Design review of the part shown in the three views and the two pictorial views. Dimensions are in mm from the part's minimum x, y and z. Round coordinates to 2 decimals unless told otherwise and drop trailing zeros. Loops run counter-clockwise (first coordinate to the right, second up) from the corner with the lowest first, then second, coordinate; pieces in that order, holes last. Notation, with made-up numbers: (-29.75, 33) -> (6.25, 33) arc R20 cw to (6.25, 55) -> close; hole circle Ø11 at (-2, 30.5). An arc over 180 degrees is marked (long way). Return JSON: item names as keys, results as strings. Group by question number.
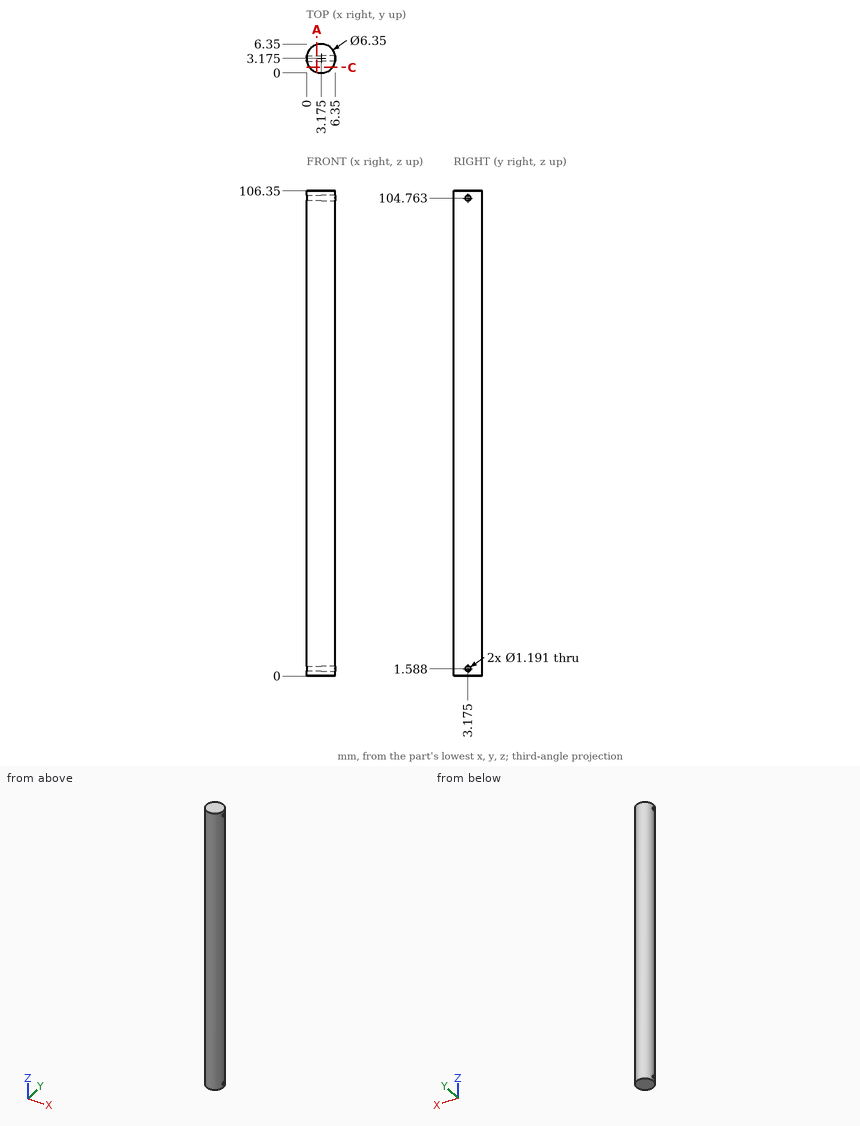
1. We need section A-A, the plane x = 2.25. Give the number of separate pieces and of enclosed holes in the cut face, then the cut area to 3 significant figures.
2. For P1, Ø1.5, axis at x = 5, z = 90, coming from the +Y side; P2, Ø1, axis at x = 1.5, z = 61.5, coming from the +Y side (1 decimal); P3, Ø1, axis at y = 3.18, z = 104.76, coming from the -X side; P4, Ø1, axis at x = 4, z = 16, coming from the -Y side, all flat-tipped, find the tip position at first contact; note any pin that passes through.
3. We need section C-C, the plane y = 1.25. Write out the cut boundary in (x, z), then the cut area to 3 significant figures.
4. Wall thickness on line 1 (X direction, y = 3.5, z = 65.5); line 2 (X direction, y = 5, z = 40) (1 decimal); line 3 (Y direction, x = 3.25, z = 81): over which ranges is each line inside the solid? List them lowest first.
Check sheet entries:
{
 "1": {"separate pieces": "1", "enclosed holes": "2", "area": "644 mm²"},
 "2": {"P1": "stops at y = 6.16", "P2": "stops at y = 6.1", "P3": "passes through", "P4": "stops at y = 0.02"},
 "3": {"outline": "(0.65, 0) -> (5.7, 0) -> (5.7, 106.35) -> (0.65, 106.35) -> close", "area": "537 mm²"},
 "4": {"line 1": "x = 0.02 to 6.33", "line 2": "x = 0.6 to 5.8", "line 3": "y = 0 to 6.35"}
}
